Here's the drawing with two shaded views (mm, measured from the low corner). I have some questions. Coordinates: 2 decimals unless noted, no trailing zeros. Loops run counter-clockwise (first coordinate to the right, second up) from the corner with the lowest first, then second, coordinate; pieces in that order, holes last. Notation, with made-up numbers: (-10, 24.5) -> (29, 24.5) arc R4 ccw to (29, 31.5) -> close; hole circle Ø3 at (-21, -11). An arc over 180 degrees is marked (long way). Use CSV: the item, a comma, the result in double quotes. Start each with the question number.
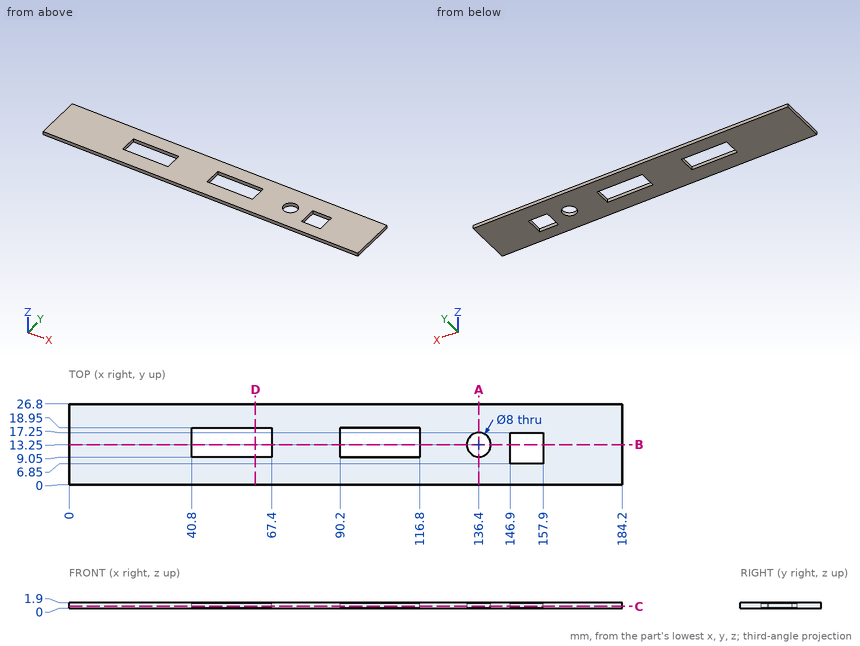
1) Please list where these lines run through material, in increasing order: L1, parallel to X at y = 13.5, z = 1.8; L2, parallel to Y at x = 136.5, z = 0.4; L3, parallel to Y at x = 151, z = 0.6. Write a range as [from, to].
2) I want a section at A-A, the plane x = 136.4. Please give me the cut outline in (y, z).
3) For P1, Ø5, axis at x = 136.4, y = 13.25, coming from the +Z side, with a flat end and sliding along its axis, tell me the tip position at first contact or that it passes through.
4) I want a section at C-C, the plane z = 0.6. Please give me the cut outline in (x, y).
5) I want a section at B-B, the plane y = 13.25. Please give me the cut outline in (x, z), plus the area to 3 significant figures.
6) I want a section at D-D, the plane x = 62. Please give me the cut outline in (y, z).
Return value:
1,L1,"x = [0, 40.8], [67.4, 90.2], [116.8, 132.41], [140.39, 146.9], [157.9, 184.2]"
1,L2,"y = [0, 9.25], [17.25, 26.8]"
1,L3,"y = [0, 6.85], [17.25, 26.8]"
2,outline,"(0, 0) -> (9.25, 0) -> (9.25, 1.9) -> (0, 1.9) -> close; (17.25, 0) -> (26.8, 0) -> (26.8, 1.9) -> (17.25, 1.9) -> close"
3,P1,"passes through"
4,outline,"(0, 0) -> (184.2, 0) -> (184.2, 26.8) -> (0, 26.8) -> close; hole (40.8, 9.05) -> (67.4, 9.05) -> (67.4, 18.95) -> (40.8, 18.95) -> close; hole (90.2, 9.05) -> (116.8, 9.05) -> (116.8, 18.95) -> (90.2, 18.95) -> close; hole circle Ø8 at (136.4, 13.25); hole (146.9, 6.85) -> (157.9, 6.85) -> (157.9, 17.25) -> (146.9, 17.25) -> close"
5,outline,"(0, 0) -> (40.8, 0) -> (40.8, 1.9) -> (0, 1.9) -> close; (67.4, 0) -> (90.2, 0) -> (90.2, 1.9) -> (67.4, 1.9) -> close; (116.8, 0) -> (132.4, 0) -> (132.4, 1.9) -> (116.8, 1.9) -> close; (140.4, 0) -> (146.9, 0) -> (146.9, 1.9) -> (140.4, 1.9) -> close; (157.9, 0) -> (184.2, 0) -> (184.2, 1.9) -> (157.9, 1.9) -> close"
5,area,"213 mm²"
6,outline,"(0, 0) -> (9.05, 0) -> (9.05, 1.9) -> (0, 1.9) -> close; (18.95, 0) -> (26.8, 0) -> (26.8, 1.9) -> (18.95, 1.9) -> close"
